Autodesk Inventor part; units mm, degrees
ref_plane "YZ Plane" through (0, 0, 0) normal (1, 0, 0) x (0, 1, 0)
ref_plane "XZ Plane" through (0, 0, 0) normal (0, 1, 0) x (-1, 0, 0)
ref_plane "XY Plane" through (0, 0, 0) normal (0, 0, 1) x (1, 0, 0)
sketch "Sketch1" plane through (0, 0, 0) normal (0, 0, 1) x (1, 0, 0)
  line L0 (-12.7, -6.35) -> (12.7, -6.35)
  line L1 (12.7, -6.35) -> (12.7, 6.35)
  line L2 (12.7, 6.35) -> (-12.7, 6.35)
  line L3 (-12.7, 6.35) -> (-12.7, -6.35)
  line L4 (-12.7, -6.35) -> (12.7, 6.35) construction
  line L5 (12.7, -6.35) -> (-12.7, 6.35) construction
  line L6 (-9.525, -3.175) -> (9.525, -3.175)
  line L7 (9.525, -3.175) -> (9.525, 3.175)
  line L8 (9.525, 3.175) -> (-9.525, 3.175)
  line L9 (-9.525, 3.175) -> (-9.525, -3.175)
  line L10 (-9.525, -3.175) -> (9.525, 3.175) construction
  line L11 (9.525, -3.175) -> (-9.525, 3.175) construction
  point P0 (0, 0)
  dimension "d0" = 25.4
  dimension "d1" = 12.7
  dimension "d2" = 3.175
  dimension "d3" = 3.175
extrude "Extrusion1" add sketch "Sketch1" along normal mid plane 334.137
sketch "Sketch2" plane through (-12.7, -6.35, 167.0685) normal (0, -1, 0) x (1, 0, 0)
  line L0 (25.4, -334.137) -> (0, -334.137)
  line L1 (25.4, -334.137) -> (0, -319.4723)
  line L2 (0, 0) -> (0, -334.137)
  line L3 (0, -334.137) -> (0, -319.4723)
  line L4 (0, -334.137) -> (25.4, -334.137)
  line L5 (22.225, -334.137) -> (22.225, 0)
  point P0 (12.7, -167.0685)
  dimension "d6" = 30
extrude "Extrusion2" cut sketch "Sketch2" against normal through all
properties part number "1x0_5x12-aluminumExtrusion" material "Aluminum 6061, Welded"
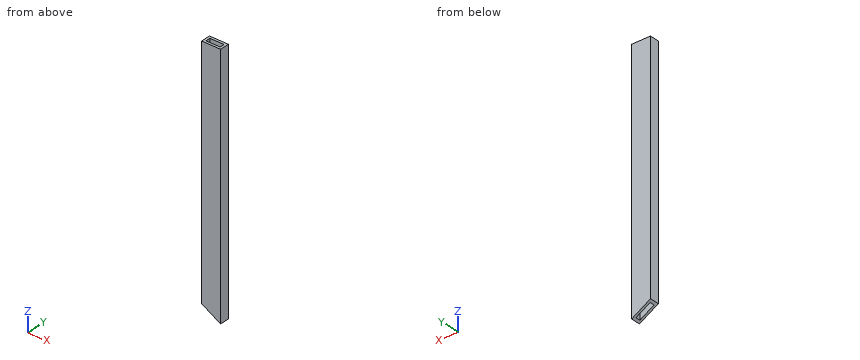
For this review, take the finished solid that the model builds, in its own axes (mm). Give positions to 0.01 mm unless a question says otherwise; leave off trailing zeros. Write each loop counter-clockwise with the first axis right and the second up, starting at its lowest first coordinate (ties: lowest second). Pieces come first, ordered by that corner, then holes.
Item 1: Wall thickness on probe 1 along X at (y, z) = (-0.75, -6) (3 decimals); probe 2 along Y at (x, z) = (3.25, -50) (3 decimals); probe 3 along Z at (x, y) = (9.5, 5): over which ranges is each line inside the solid? List them lowest first.
Item 2: Take a section at C-C (z = -16.5). Give the boundary of the cut face in (x, y) (3 decimals).
Item 3: Take a section at A-A (y = -1.25). Give the boundary of the cut face in (x, z) (1 decimal).
Item 4: Insertion check: P1, Ø3, axis at x = -5, y = -1.5, coming from the +Z side; P2, Ø1, axis at x = 4.5, y = -5, coming from the -Z side. Each pin has a flat end and moves straight along its axis. Give the tip position at first contact, or say it passes through.
Established:
1. probe 1: x = -12.7 to -9.525, 9.525 to 12.7
1. probe 2: y = -6.35 to -3.175, 3.175 to 6.35
1. probe 3: z = -165.22 to 167.07
2. outline: (-12.7, -6.35) - (12.7, -6.35) - (12.7, 6.35) - (-12.7, 6.35) - close; hole (-9.525, -3.175) - (9.525, -3.175) - (9.525, 3.175) - (-9.525, 3.175) - close
3. outline: (-12.7, -152.4) - (-9.5, -154.2) - (-9.5, 167.1) - (-12.7, 167.1) - close; (9.5, -165.2) - (12.7, -167.1) - (12.7, 167.1) - (9.5, 167.1) - close
4. P1: passes through
4. P2: stops at z = -162.62
